```python
from build123d import *

# Parameters (mm, degrees)
BOSS_EXTRUDE1_DEPTH = 50
SKETCH2_R           = 1.516102493
CUT_EXTRUDE1_DEPTH  = 10
SKETCH3_R           = 1.505855903
BOSS_EXTRUDE2_DEPTH = 5


with BuildPart() as part:
    # Sketch1 → Boss-Extrude1 (new body)
    with BuildSketch(Plane(origin=(0, 0, 0), x_dir=(1, 0, 0), z_dir=(0, 1, 0))):
        Polygon((0, -2.886751346), (2.5, -1.443375673), (2.5, 1.443375673), (0, 2.886751346), (-2.5, 1.443375673), (-2.5, -1.443375673), align=None)
    extrude(amount=BOSS_EXTRUDE1_DEPTH)

    # Sketch2 → Cut-Extrude1 (cut)
    with BuildSketch(Plane(origin=(0, 50, 0), x_dir=(1, 0, 0), z_dir=(0, 1, 0))):
        Circle(SKETCH2_R)
    extrude(amount=-CUT_EXTRUDE1_DEPTH, mode=Mode.SUBTRACT)

    # Sketch3 → Boss-Extrude2 (add)
    with BuildSketch(Plane.XZ):
        Circle(SKETCH3_R)
    extrude(amount=BOSS_EXTRUDE2_DEPTH)


solid = part.part
```
Verification items for the finished model (mm, model axes). A direction names the side the tool comes from. Round coordinates to 2 decimals unless told otherwise and drop trailing zeros. Write each loop counter-clockwise with the first axis right and the second up, starting at its lowest first coordinate (ties: lowest second). Pieces come first, ordered by that corner, then holes.
1. Draft check along Z on faces 1 (the flat face through (0, 40, 0)), 2 (the flat face through (2.5, 25, 0)), 3 (the cylindrical face through (-1.515, 45.07, -0.067)), 4 (the flat face through (-1.267, 24.65, 2.155)). Enter one of: +Z half, -Z half, draft (parallel to the pull), parting line (faces both ways), or undercut.
2. Section check D-D on y = -1. Enter the section's corners in (x, z), plus the area to 3 significant figures.
3. Section check B-B on y = 33. Enter the section's corners in (x, z), plus the area to 3 significant figures.
4. Gauge pin test, flat ends, axial feed: P1, Ø3, axis at x = -2, y = 20, coming from the -Z side; P2, Ø1.5, axis at x = -0.5, y = 20, coming from the +Z side; P3, Ø0.9, axis at x = -0.5, z = 0.5, coming from the +Y side. Record the tip position at first contact, or that the pin passes through.
5. Scan lines: L1, parallel to X at y = 45.75, z = 0; L2, parallel to Z at x = 0, y = 45.75; L3, parallel to Y at x = 2.15, z = -0.8. Record each from-to range of solid material in increasing order.
6. Access from +Z, -Z, +X, -X, +Y, -Y to the whole of each face (thin tool, end or side, straight path). Record for faces 5 (the flat face through (0, -5, 0)), 6 (the flat face through (-1.15, 0, 1.24)).
7. Section check A-A on z = 0. Enter the section's corners in (x, y).
8. Section check C-C on x = -0.8. Enter the section's corners in (y, z), plus the area to 3 significant figures.
Answer:
1. face 1: undercut
1. face 2: draft
1. face 3: undercut
1. face 4: +Z half
2. outline: circle Ø3.01 at (0, 0)
2. area: 7.12 mm2
3. outline: (-2.5, -1.44) - (0, -2.89) - (2.5, -1.44) - (2.5, 1.44) - (0, 2.89) - (-2.5, 1.44) - close
3. area: 21.7 mm2
4. P1: stops at z = -2.6
4. P2: stops at z = 2.89
4. P3: stops at y = 40
5. L1: x = -2.5 to -1.52, 1.52 to 2.5
5. L2: z = -2.89 to -1.52, 1.52 to 2.89
5. L3: y = 0 to 50
6. face 5: +Z, -Z, +X, -X, -Y
6. face 6: -Y
7. outline: (-2.5, 0) - (-1.51, 0) - (-1.51, -5) - (1.51, -5) - (1.51, 0) - (2.5, 0) - (2.5, 50) - (1.52, 50) - (1.52, 40) - (-1.52, 40) - (-1.52, 50) - (-2.5, 50) - close
8. outline: (-5, -1.28) - (0, -1.28) - (0, -2.42) - (50, -2.42) - (50, -1.29) - (40, -1.29) - (40, 1.29) - (50, 1.29) - (50, 2.42) - (0, 2.42) - (0, 1.28) - (-5, 1.28) - close
8. area: 229 mm2
